Can you work these out from the drawing? Everything is in mm from the part's minimum corner. A direction names the side the tool comes from. Give positions to 0.01 mm unless a question says otherwise; leave off trailing zeros. Write each loop counter-clockwise with the first axis right and the second up, starting at its lowest first coordinate (ties: lowest second). Pieces come first, ordered by that corner, then holes. Notation, with made-up numbers: M 12.5,81.5 L 51.5,81.5 A23 ccw 51.5,120.5 Z; hole C -15,67 d10. An arc over 180 degrees is marked long. One line per item, written item: value.
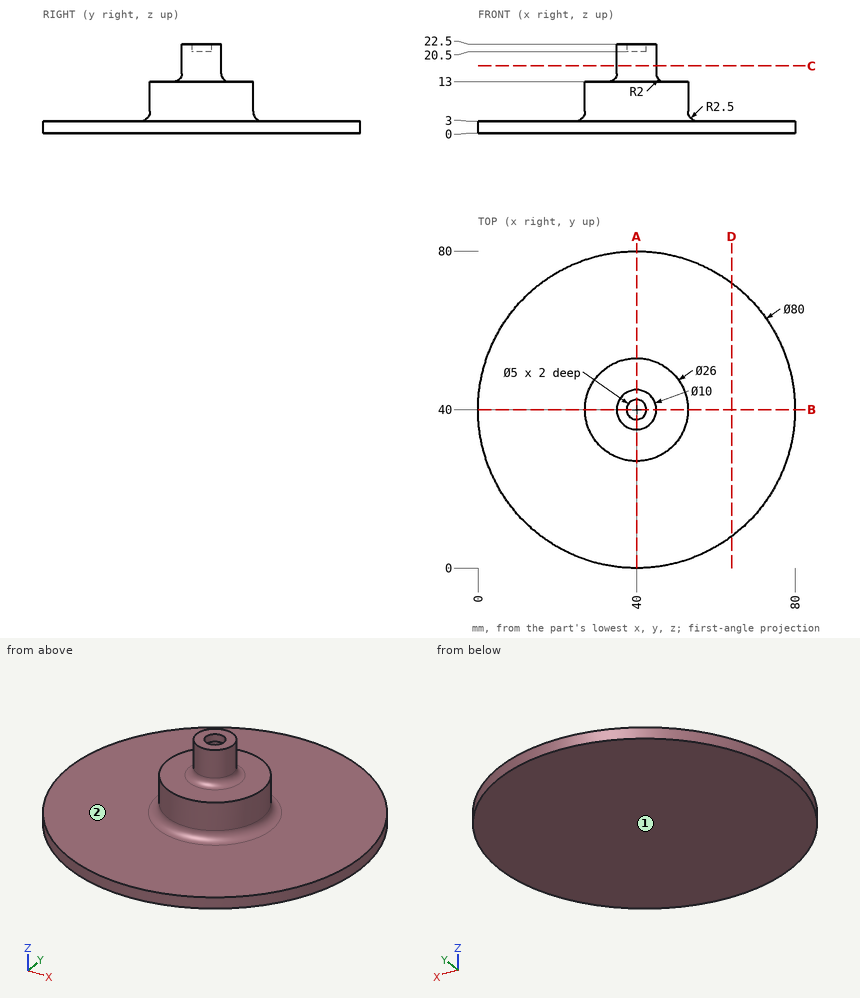
1) Please list where these lines run through material, in increasing order: L1, parallel to Y at x = 40, z = 21.25; L2, parallel to Z at x = 60.5, y = 36; L3, parallel to Y at x = 50, z = 10.5. Write a range as from..to.
Outcome:
L1: y = 35..37.5, 42.5..45
L2: z = 0..3
L3: y = 31.69..48.31
2) If we section it at D-D, the plane x = 64: Write out the boundary of the cut face in (y, z), then the cut area to 3 significant figures.
Outcome:
outline: M 8,0 L 72,0 L 72,3 L 8,3 Z
area: 192 mm^2
3) If we section it at C-C, the plane z = 17: Write out the boundary of the cut face in (x, y).
Outcome:
outline: C 40,40 d10
4) If we section it at A-A, the plane x = 40: Write out the boundary of the cut face in (y, z), then the cut area to 3 significant figures.
Outcome:
outline: M 0,0 L 80,0 L 80,3 L 55.5,3 A2.5 cw 53,5.5 L 53,13 L 47,13 A2 cw 45,15 L 45,22.5 L 42.5,22.5 L 42.5,20.5 L 37.5,20.5 L 37.5,22.5 L 35,22.5 L 35,15 A2 cw 33,13 L 27,13 L 27,5.5 A2.5 cw 24.5,3 L 0,3 Z
area: 589 mm^2
5) On a 3-axis mill with a long thin cutter (end or side, diameter ignored), from which of +Z, -Z, +X, -X, +Y, -Y can I reach the whole of each face in a straight line? I mean the marked faces 1 and 2. Say none if no direction works.
Outcome:
face 1: -Z, +X, -X, +Y, -Y
face 2: +Z
6) I'm going to push flat-ended pins straight in: pin 1 (4 mm diameter, centred on x = 37.5, y = 50, fed in from +Z); pin 2 (24 mm diameter, centred on x = 30.5, y = 43, fed in from +Z); pin 3 (2 mm diameter, centred on x = 55, y = 49.5, fed in from +Z). Where does each tip first touch, or does it pass through?
Outcome:
pin 1: stops at z = 13
pin 2: stops at z = 22.5
pin 3: stops at z = 3
